Design review of the part built by this model. Coordinates are the model's own, in mm. A direction names the side the tool comes from. Coordinates: 2 decimals unless noted, no trailing zeros. Order: outer loops, then holes, each group sorted by start corner. A loop starts at its lowest first (then second) coordinate and runs counter-clockwise, first axis right, second up. Notation, with made-up numbers: (-7.75, 51.5) - (11.25, 51.5) arc R19 cw to (11.25, 57.5) - close; hole circle Ø2 at (79.5, 72). An arc over 180 degrees is marked (long way). Write item = value, one per line. Start each with the question number.
```python
from build123d import *

# Parameters (mm, degrees)
EXTRUDE_1_DEPTH = 3
SKETCH_2_R      = 5.5
EXTRUDE_2_DEPTH = 1.5


with BuildPart() as part:
    # 草图1 → 凸台-拉伸1 (new body)
    with BuildSketch(Plane(origin=(0, 0, 0), x_dir=(1, 0, 0), z_dir=(0, 1, 0))):
        with BuildLine():
            Line((-13.570297544, 2.4), (-8.570297544, 2.4))
            ThreePointArc((-8.570297544, 2.4), (-6.293250353, 6.293250353), (-2.4, 8.570297544))
            Line((-2.4, 8.570297544), (-2.4, 13.570297544))
            Line((-2.4, 13.570297544), (2.4, 13.570297544))
            Line((2.4, 13.570297544), (2.4, 8.570297544))
            ThreePointArc((2.4, 8.570297544), (6.293250353, 6.293250353), (8.570297544, 2.4))
            Line((8.570297544, 2.4), (13.570297544, 2.4))
            Line((13.570297544, 2.4), (13.570297544, -2.4))
            Line((13.570297544, -2.4), (8.570297544, -2.4))
            ThreePointArc((8.570297544, -2.4), (6.293250353, -6.293250353), (2.4, -8.570297544))
            Line((2.4, -8.570297544), (2.4, -13.570297544))
            Line((2.4, -13.570297544), (-2.4, -13.570297544))
            Line((-2.4, -13.570297544), (-2.4, -8.570297544))
            ThreePointArc((-2.4, -8.570297544), (-6.293250353, -6.293250353), (-8.570297544, -2.4))
            Line((-8.570297544, -2.4), (-13.570297544, -2.4))
            Line((-13.570297544, -2.4), (-13.570297544, 2.4))
        make_face()
    extrude(amount=EXTRUDE_1_DEPTH)

    # 草图2 → 凸台-拉伸2 (add)
    with BuildSketch(Plane(origin=(0, 3, 0), x_dir=(1, 0, 0), z_dir=(0, 1, 0))):
        Circle(SKETCH_2_R)
    extrude(amount=EXTRUDE_2_DEPTH)


solid = part.part
```
Item 1: For P1, Ø0.9, axis at x = -10.5, y = 1.5, coming from the -Z side; P2, Ø2, axis at y = 3, z = 10, coming from the +X side; P3, Ø0.9, axis at x = 12, y = 1.5, coming from the +Z side; P4, Ø1.5, axis at x = 5, z = -9, coming from the +Y side, all flat-tipped, find the tip position at first contact; note any pin that passes through.
Item 2: Add section C-C on x = 0. Give the boundary of the cut face in (y, z).
Item 3: Add section D-D on x = -10.5. Give the boundary of the cut face in (y, z).
Item 4: Add section A-A on y = 0.4. Give the boundary of the cut face in (x, z).
Item 5: For faces 1 (the flat face through (4, 3, -4)), 2 (the flat face through (2.4, 1, -11)), 3 (the flat face through (-2.4, 1, 11)), 4 (the flat face through (2.4, 1, 11)), 5 (the flat face through (-11, 1, -2.4)), list the 3-axis set-ups (+Z, -Z, +X, -X, +Y, -Y) from which the entire face can be reached by the end or side of a thin tool; tool diameter is ignored.
Item 6: For line 1 (X direction, y = 0.5, z = 10.5); line 2 (Y direction, x = -3.5, z = 7.5), list the stretches that pass through material, from the lowest coordinate up.
Item 7: Add section B-B on z = 0. Give the boundary of the cut face in (x, y), plus the area to 3 significant figures.
Worked out:
q1.P1 = -2.4
q1.P2 = 2.4
q1.P3 = 2.4
q1.P4 = through
q2.outline = (0, -13.57) - (3, -13.57) - (3, -5.5) - (4.5, -5.5) - (4.5, 5.5) - (3, 5.5) - (3, 13.57) - (0, 13.57) - close
q3.outline = (0, -2.4) - (3, -2.4) - (3, 2.4) - (0, 2.4) - close
q4.outline = (-13.57, -2.4) - (-8.57, -2.4) arc R8.9 ccw to (-2.4, -8.57) - (-2.4, -13.57) - (2.4, -13.57) - (2.4, -8.57) arc R8.9 ccw to (8.57, -2.4) - (13.57, -2.4) - (13.57, 2.4) - (8.57, 2.4) arc R8.9 ccw to (2.4, 8.57) - (2.4, 13.57) - (-2.4, 13.57) - (-2.4, 8.57) arc R8.9 ccw to (-8.57, 2.4) - (-13.57, 2.4) - close
q5.face_1 = +Y
q5.face_2 = -Z, +X, +Y, -Y
q5.face_3 = +Z, -X, +Y, -Y
q5.face_4 = +Z, +X, +Y, -Y
q5.face_5 = -Z, -X, +Y, -Y
q6.line_1 = -2.4 to 2.4
q6.line_2 = 0 to 3
q7.outline = (-13.57, 0) - (13.57, 0) - (13.57, 3) - (5.5, 3) - (5.5, 4.5) - (-5.5, 4.5) - (-5.5, 3) - (-13.57, 3) - close
q7.area = 97.9 mm2
